Autodesk Fusion 360 part; units mm, degrees
sketch "Sketch1" plane through (0, 0, 0) normal (0, 1, 0) x (1, 0, 0)
  circle A0 centre (0, 0) radius 3
  circle A1 centre (0, 0) radius 5
  line L0 (0, 0) -> (-50, 0) construction
  circle A2 centre (-50, 0) radius 3
  circle A3 centre (-50, 0) radius 5
  line L1 (-50, -5) -> (0, -5)
  line L2 (0, 5) -> (-50, 5)
  dimension "d1" = 6
  dimension "d2" = 10
  dimension "d3" = 50
  dimension "d4" = 6
  dimension "d5" = 10
extrude "Extrude1" add sketch "Sketch1" along normal blind 10
sketch "Sketch2" plane through (0, 10, 0) normal (0, 1, 0) x (-1, 0, 0)
  circle A0 centre (50, 0) radius 3
  circle A1 centre (0, 0) radius 3
  line L0 (0, -5) -> (50, -5)
  arc A2 (50, -5) -> (50, 5) centre (50, 0) ccw
  line L1 (50, 5) -> (0, 5)
  arc A3 (0, 5) -> (0, -5) centre (0, 0) ccw
  line L2 (11, 5) -> (39, 5)
  line L3 (39, 5) -> (39, -5)
  line L4 (39, -5) -> (11, -5)
  line L5 (11, -5) -> (11, 5)
  dimension "d8" = 28
extrude "Extrude2" add sketch "Sketch2" along normal blind 40 contours L0 L1 L2 L3 L4 L5
sketch "Sketch3" plane through (0, 0, 5) normal (0, 0, 1) x (-1, 0, 0)
  line L0 (50, 0) -> (0, 0)
  line L1 (0, 0) -> (0, -10)
  line L2 (0, -10) -> (11, -10)
  line L3 (11, -10) -> (11, -50)
  line L4 (11, -50) -> (39, -50)
  line L5 (39, -50) -> (39, -10)
  line L6 (39, -10) -> (50, -10)
  line L7 (50, -10) -> (50, 0)
  line L8 (11, -10) -> (39, -10) construction
  line L9 (25, -10) -> (25, -15) construction
  line L10 (34, -45.5) -> (16, -45.5)
  line L11 (16, -45.5) -> (16, -15)
  line L12 (16, -15) -> (34, -15)
  line L13 (34, -15) -> (34, -45.5)
  dimension "d11" = 5
  dimension "d12" = 18
  dimension "d13" = 30.5
extrude "Extrude3" cut sketch "Sketch3" against normal blind 10 contours L10 L11 L12 L13
Read the model definition and answer for the solid it produces. Units are mm, in the model's axes. A direction names the side the tool comes from. Give positions to 0.01 mm unless a question says otherwise; leave off trailing zeros. Order: outer loops, then holes, each group sorted by start corner. A loop starts at its lowest first (then second) coordinate and runs counter-clockwise, first axis right, second up. Notation, with made-up numbers: (-21, 6) -> (-9, 6) arc R9 ccw to (-9, 18) -> close; hole circle Ø2 at (66.5, 24). An arc over 180 degrees is marked (long way). One line per item, written item: value. Start each with the question number.
(1) For a pull along Z with two mould halves and no side action, classify faces 6 (the flat face through (-25, 50, 0)), 7 (the cylindrical face through (-3, 5, 0)), 8 (the cylindrical face through (5, 5, 0)) as released by +Z, released by -Z, zero draft, split by the parting line, or undercut.
(2) The part is cut by section B-B (x = -33). Determine the outline of the cut face in (y, z).
(3) Flat-ended cylindrical pins translate along their axes: P1, Ø1, axis at y = 17.5, z = 4, coming from the +X side; P2, Ø3, axis at y = 7, z = 4, coming from the +X side; P3, Ø3, axis at y = 35.5, z = -1, coming from the -X side. Find the tip coordinate at first contact, or state that the pin passes through.
(4) The part is cut by section A-A (z = 0). Determine the outline of the cut face in (x, y), and give its area (3 significant figures).
(5) The part is cut by section D-D (z = 4). Determine the outline of the cut face in (x, y).
(6) A tool of negligible diameter and unlimited length cuts with its end or side. For faces 1 (the flat face through (-25, 14, 5)), 2 (the cylindrical face through (-55, 5, 0)), 3 (the flat face through (-5, 10, 0)), 4 (the flat face through (-16, 30, 0)), 5 (the flat face through (-45, 10, 0)), from which of +Z, -Z, +X, -X, +Y, -Y can it reach the whole face along a straight path? Write none if from no direction.
(7) Straight lines are drawn through the part: L1, parallel to X at y = 4.5, z = 0; L2, parallel to Y at x = -29, z = -3; L3, parallel to X at y = 21, z = 1.75. For each, find the intervals that lie inside material, in ascending order.
(8) The part is cut by section C-C (y = 37.5). Determine the outline of the cut face in (x, z), and give its area (3 significant figures).
Taken from the geometry:
1. face 6: zero draft
1. face 7: undercut
1. face 8: split by the parting line
2. outline: (0, -5) -> (15, -5) -> (15, 5) -> (0, 5) -> close; (45.5, -5) -> (50, -5) -> (50, 5) -> (45.5, 5) -> close
3. P1: x = -11
3. P2: x = 4.33
3. P3: x = -39
4. outline: (-55, 0) -> (-53, 0) -> (-53, 10) -> (-55, 10) -> close; (-47, 0) -> (-3, 0) -> (-3, 10) -> (-11, 10) -> (-11, 50) -> (-39, 50) -> (-39, 10) -> (-47, 10) -> close; (3, 0) -> (5, 0) -> (5, 10) -> (3, 10) -> close; hole (-34, 15) -> (-16, 15) -> (-16, 45.5) -> (-34, 45.5) -> close
4. area: 1,050 mm^2
5. outline: (-53, 0) -> (3, 0) -> (3, 10) -> (-11, 10) -> (-11, 50) -> (-39, 50) -> (-39, 10) -> (-53, 10) -> close; hole (-34, 15) -> (-16, 15) -> (-16, 45.5) -> (-34, 45.5) -> close
6. face 1: +Z, +X, -X, +Y, -Y
6. face 2: -X, +Y, -Y
6. face 3: +Z, -Z, +X, +Y
6. face 4: +Z, -Z
6. face 5: +Z, -Z, -X, +Y
7. L1: -55 to -53, -47 to -3, 3 to 5
7. L2: 0 to 15, 45.5 to 50
7. L3: -39 to -34, -16 to -11
8. outline: (-39, -5) -> (-34, -5) -> (-34, 5) -> (-39, 5) -> close; (-16, -5) -> (-11, -5) -> (-11, 5) -> (-16, 5) -> close
8. area: 100 mm^2
